Verification items for the finished model (mm, model axes). Give positions to 0.01 mm unless a question says otherwise; leave off trailing zeros. Order: outer loops, then holes, each group sorted by start corner. A loop starts at its lowest first (then second) coordinate and runs counter-clockwise, first axis right, second up. Notation, with made-up numbers: (50, -15.75) -> (107, -15.75) arc R17 ccw to (107, 10.25) -> close; hole circle Ø1 at (-29.75, 45.5). An arc over 180 degrees is marked (long way). One line per question, with ' | ' between items. Start each with the question number.
Q1. Material ranges on probe 1 along Z at (x, y) = (-40, 1.75); probe 2 along X at (y, z) = (3.5, -41.5); probe 3 along Z at (x, y) = (5, 2.5), recorded low to high. Write a range as [from, to].
Q2. Section check C-C on x = -13. Record the cut outline in (y, z).
Q3. Section check A-A on z = -5. Record the cut outline in (x, y).
Q4. Section check B-B on x = -3. Record the cut outline in (y, z), plus the area to 3 significant figures.
Q5. Section check D-D on y = 1.75. Give the number of separate pieces and of enclosed holes in the cut face, plus the area to 3 significant figures.
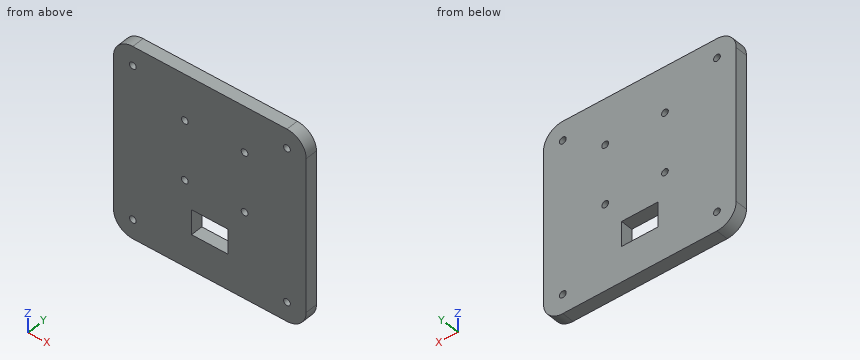
from build123d import *

# Parameters (mm, degrees)
SKETCH2_W                 = 100
SKETCH2_H                 = 100
BOSS_EXTRUDE1_DEPTH       = 6.35
SKETCH3_R                 = 1.75
CUT_EXTRUDE1_DEPTH        = 7.35
LPATTERN1_COUNT           = 2
LPATTERN1_PITCH           = 80
LPATTERN2_COUNT           = 2
LPATTERN2_PITCH           = 80
LPATTERN2_COPY_1_SKETCH_R = 1.75
LPATTERN2_COPY_1_DEPTH    = 7.35
SKETCH8_R                 = 1.75
CUT_EXTRUDE2_DEPTH        = 7.35
LPATTERN3_COUNT           = 2
LPATTERN3_PITCH           = 31
LPATTERN4_COUNT           = 2
LPATTERN4_PITCH           = 31
LPATTERN4_COPY_1_SKETCH_R = 1.75
LPATTERN4_COPY_1_DEPTH    = 7.35
SKETCH9_W                 = 19
SKETCH9_H                 = 13
CUT_EXTRUDE3_DEPTH        = 7.35
FILLET1_R                 = 10


with BuildPart() as part:
    # Sketch2 → Boss-Extrude1 (new body)
    with BuildSketch(Plane(origin=(0, 0, 0), x_dir=(1, 0, 0), z_dir=(0, 1, 0))):
        Rectangle(SKETCH2_W, SKETCH2_H)
    extrude(amount=BOSS_EXTRUDE1_DEPTH)

    # Sketch3 → Cut-Extrude1 (cut, through all)
    with BuildSketch(Plane.XZ):
        with Locations((-40, -40)):
            Circle(SKETCH3_R)
    cut_extrude1 = extrude(amount=-CUT_EXTRUDE1_DEPTH, mode=Mode.SUBTRACT)

    # LPattern1: Cut-Extrude1 ×2
    with Locations(*[(0, 0, i * LPATTERN1_PITCH) for i in range(1, LPATTERN1_COUNT)]):
        add(cut_extrude1, mode=Mode.SUBTRACT)

    # LPattern2: Cut-Extrude1 ×2
    with Locations(*[(i * LPATTERN2_PITCH, 0, 0) for i in range(1, LPATTERN2_COUNT)]):
        add(cut_extrude1, mode=Mode.SUBTRACT)

    # LPattern2 copy 1 sketch → LPattern2 copy 1 (cut, through all)
    with BuildSketch(Plane(origin=(80, 0, 80), x_dir=(1, 0, 0), z_dir=(0, -1, 0))):
        with Locations((-40, -40)):
            Circle(LPATTERN2_COPY_1_SKETCH_R)
    extrude(amount=-LPATTERN2_COPY_1_DEPTH, mode=Mode.SUBTRACT)

    # Sketch8 → Cut-Extrude2 (cut, through all)
    with BuildSketch(Plane.XZ):
        with Locations((18, -5)):
            Circle(SKETCH8_R)
    cut_extrude2 = extrude(amount=-CUT_EXTRUDE2_DEPTH, mode=Mode.SUBTRACT)

    # LPattern3: Cut-Extrude2 ×2
    with Locations(*[(0, 0, i * LPATTERN3_PITCH) for i in range(1, LPATTERN3_COUNT)]):
        add(cut_extrude2, mode=Mode.SUBTRACT)

    # LPattern4: Cut-Extrude2 ×2
    with Locations(*[(-i * LPATTERN4_PITCH, 0, 0) for i in range(1, LPATTERN4_COUNT)]):
        add(cut_extrude2, mode=Mode.SUBTRACT)

    # LPattern4 copy 1 sketch → LPattern4 copy 1 (cut, through all)
    with BuildSketch(Plane(origin=(-31, 0, 31), x_dir=(1, 0, 0), z_dir=(0, -1, 0))):
        with Locations((18, -5)):
            Circle(LPATTERN4_COPY_1_SKETCH_R)
    extrude(amount=-LPATTERN4_COPY_1_DEPTH, mode=Mode.SUBTRACT)

    # Sketch9 → Cut-Extrude3 (cut, through all)
    with BuildSketch(Plane.XZ):
        with Locations((0, -25)):
            Rectangle(SKETCH9_W, SKETCH9_H)
    extrude(amount=-CUT_EXTRUDE3_DEPTH, mode=Mode.SUBTRACT)

    # Fillet1
    fillet1_edges = [part.edges().sort_by_distance(p)[0] for p in [
        (-50, 3.175, -50),
        (-50, 3.175, 50),
        (50, 3.175, 50),
        (50, 3.175, -50),
    ]]
    fillet(fillet1_edges, radius=FILLET1_R)


solid = part.part
Filled in:
1) probe 1: [-50, -41.75], [-38.25, 38.25], [41.75, 50] | probe 2: [-49.89, -40.9], [-39.1, 39.1], [40.9, 49.89] | probe 3: [-50, -31.5], [-18.5, 50]
2) outline: (0, -50) -> (6.35, -50) -> (6.35, -6.75) -> (0, -6.75) -> close; (0, -3.25) -> (6.35, -3.25) -> (6.35, 24.25) -> (0, 24.25) -> close; (0, 27.75) -> (6.35, 27.75) -> (6.35, 50) -> (0, 50) -> close
3) outline: (-50, 0) -> (-14.75, 0) -> (-14.75, 6.35) -> (-50, 6.35) -> close; (-11.25, 0) -> (16.25, 0) -> (16.25, 6.35) -> (-11.25, 6.35) -> close; (19.75, 0) -> (50, 0) -> (50, 6.35) -> (19.75, 6.35) -> close
4) outline: (0, -50) -> (6.35, -50) -> (6.35, -31.5) -> (0, -31.5) -> close; (0, -18.5) -> (6.35, -18.5) -> (6.35, 50) -> (0, 50) -> close | area: 552 mm²
5) separate pieces: 1 | enclosed holes: 9 | area: 9,590 mm²
